Autodesk Inventor part; units mm, degrees
ref_plane "YZ Plane" through (0, 0, 0) normal (1, 0, 0) x (0, 1, 0)
ref_plane "XZ Plane" through (0, 0, 0) normal (0, 1, 0) x (-1, 0, 0)
ref_plane "XY Plane" through (0, 0, 0) normal (0, 0, 1) x (1, 0, 0)
sketch "Sketch1" plane through (0, 0, 0) normal (0, 1, 0) x (-1, 0, 0)
  line L0 (0, 0) -> (-70, 0)
  line L1 (-70, 0) -> (-70, 165)
  line L2 (-70, 165) -> (0, 165)
  line L3 (0, 165) -> (0, 0)
  dimension "d0" = 70
  dimension "d1" = 165
extrude "Extrusion1" add sketch "Sketch1" along normal blind 7
sketch "Sketch2" plane through (0, 0, 0) normal (0, -1, 0) x (1, 0, 0)
  line L0 (70, 165) -> (70, 0)
  line L1 (70, 0) -> (55, 0)
  line L2 (55, 0) -> (55, 15.9792)
  line L3 (55, 15.9792) -> (70, 15.9792)
  line L4 (70, 15.9792) -> (70, 0)
  line L5 (70, 0) -> (0, 0)
  line L6 (0, 0) -> (15, 0)
  line L7 (15, 0) -> (15, 13.5714)
  line L8 (15, 13.5714) -> (0, 13.5714)
  line L9 (0, 13.5714) -> (0, 0)
  line L10 (70, 165.2646) -> (55, 165.2646)
  line L11 (55, 165.2646) -> (55, 149.7232)
  line L12 (55, 149.7232) -> (70, 149.7232)
  line L13 (70, 149.7232) -> (70, 165.2646)
  line L14 (0, 165.2646) -> (15, 165.2646)
  line L15 (15, 165.2646) -> (15, 148.1909)
  line L16 (15, 148.1909) -> (0, 148.1909)
  line L17 (0, 148.1909) -> (0, 165.2646)
  line L18 (68, 151.7232) -> (57, 151.7232)
  line L19 (57, 151.7232) -> (57, 163.2646)
  line L20 (57, 163.2646) -> (68, 163.2646)
  line L21 (68, 163.2646) -> (68, 151.7232)
  line L22 (2, 150.1909) -> (13, 150.1909)
  line L23 (13, 150.1909) -> (13, 163.2646)
  line L24 (13, 163.2646) -> (2, 163.2646)
  line L25 (2, 163.2646) -> (2, 150.1909)
  line L26 (2, 11.5714) -> (13, 11.5714)
  line L27 (13, 11.5714) -> (13, 2)
  line L28 (13, 2) -> (2, 2)
  line L29 (2, 2) -> (2, 11.5714)
  line L30 (68, 13.9792) -> (57, 13.9792)
  line L31 (57, 13.9792) -> (57, 2)
  line L32 (57, 2) -> (68, 2)
  line L33 (68, 2) -> (68, 13.9792)
  dimension "d4" = 15
  dimension "d5" = 15
  dimension "d6" = 15
  dimension "d7" = 15
  dimension "d8" = 2
  dimension "d9" = 2
  dimension "d10" = 2
  dimension "d11" = 2
extrude "Extrusion2" add sketch "Sketch2" along normal blind 41
sketch "Sketch8" plane through (0, 7, 0) normal (0, 1, 0) x (1, 0, 0)
  line L0 (0, 0) -> (0, -165)
  line L1 (0, -165) -> (0, -130)
  line L2 (35, -130) -> (25, -130)
  line L3 (25, -130) -> (25, -136)
  line L4 (25, -136) -> (35, -136)
  line L5 (35, -136) -> (35, -130)
  line L6 (15, -130) -> (15, -120)
  line L7 (15, -120) -> (45, -120)
  line L8 (45, -120) -> (45, -130)
  line L9 (45, -130) -> (15, -130)
  line L10 (15, -130) -> (15, -120)
  dimension "d45" = 35
  dimension "d47" = 10
  dimension "d53" = 30
extrude "Extrusion8" add sketch "Sketch8" along normal blind 2.5 contours L2 L9 L6 L7 L8
extrude "Extrusion9" cut sketch "Sketch8" against normal blind 7 contours L5 L4 L3 L2
properties part number "piano laterale"
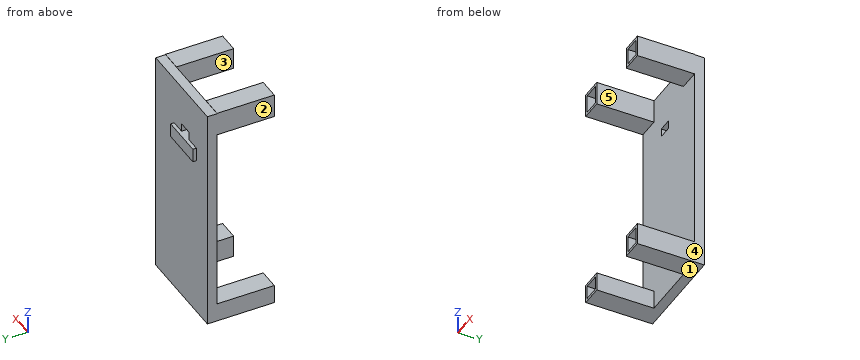
For this review, take the finished solid that the model builds, in its own axes (mm). Face numbers are marked on the shaded views. A direction names the side the tool comes from. Round coordinates to 2 decimals unless told otherwise and drop trailing zeros. Order: outer loops, then holes, each group sorted by start corner. A loop starts at its lowest first (then second) coordinate and runs counter-clockwise, first axis right, second up. Notation, with made-up numbers: (57, -31) -> (84, -31) arc R11 ccw to (84, -13) -> close; hole circle Ø8 at (17, 75). An arc over 180 degrees is marked (long way). Write item = value, one per line. Start each with the question number.
1) Take a section at A-A on y = -23.5. Count the separate pieces of the cut face and the enclosed holes in it, plus the area to 3 significant figures.
2) Take a section at B-B on x = 22.5. State the section outline as (y, z) points.
3) Take a section at C-C on z = 36. State the section outline as (x, y) points, plus the area to 3 significant figures.
4) Insertion check: pin 1 (12 mm diameter, centred on x = 60, z = 86, fed in from -Y); pin 2 (1 mm diameter, centred on x = 16, y = -17, fed in from -Z); pin 3 (5 mm diameter, centred on x = 29, y = 4.5, fed in from +Z); pin 4 (1.2 mm diameter, centred on x = 24, y = 8, fed in from -Z). Each pin has a flat end and moves straight along its axis. Give the tip position at first contact, or say it passes through.
5) Tool access review of the marked faces 4 and 5: name each direction out of +Z, -Z, +X, -X, +Y, -Y from which nothing blocks a thin tool from reaching the whole face with its end or side.
6) The part is to be moulded in two halves that separate along X. For the marked faces 1, 2 and 3, say which applies: +X half, -X half, draft (parallel to the pull), parting line (faces both ways), or undercut.
7) To check wall thickness, follow line 1 (Z direction, x = 7, y = -26); line 2 (X direction, y = -6, z = 10.5); line 3 (X direction, y = 3, z = 135). State the ranges of each line that lie inside material, in increasing order. Write a range as from..to.
Verdict:
q1.separate_pieces = 4
q1.enclosed_holes = 4
q1.area = 425 mm2
q2.outline = (0, 0) -> (7, 0) -> (7, 120) -> (9.5, 120) -> (9.5, 130) -> (7, 130) -> (7, 165) -> (0, 165) -> close
q3.outline = (0, 0) -> (70, 0) -> (70, 7) -> (0, 7) -> close
q3.area = 490 mm2
q4.pin_1 = 0
q4.pin_2 = through
q4.pin_3 = 165
q4.pin_4 = 120
q5.face_4 = +Z, -Z, +X, +Y, -Y
q5.face_5 = +Z, -Z, -Y
q6.face_1 = draft
q6.face_2 = -X half
q6.face_3 = undercut
q7.line_1 = 0..2, 11.57..13.57, 148.19..150.19, 163.26..165.26
q7.line_2 = 0..2, 13..15, 55..57, 68..70
q7.line_3 = 0..25, 35..70
